Work out the finished part from the listing and answer in its coordinate system (mm). Give positions to 0.01 mm unless a question says otherwise; leave off trailing zeros. Order: outer loops, then holes, each group sorted by start corner. A loop starts at its lowest first (then second) coordinate and runs counter-clockwise, first axis right, second up. Notation, with made-up numbers: (-4.75, -30) - (41.25, -30) arc R26 cw to (41.25, -7) - close; hole circle Ø3 at (78.5, 86). An arc over 180 degrees is marked (long way). Return JSON: item names as keys, results as strings. Group by question number.
from build123d import *

# Parameters (mm, degrees)
F0_R     = 2.49938
F1_DEPTH = 101.6


with BuildPart() as f1:
    # F0 (on Front) → F1 (new body)
    with BuildSketch(Plane.XZ):
        with BuildLine():
            ThreePointArc((-24.424371, 19.05), (-45.903919, 14.384096), (-62.524371, 0))
            Line((-62.524371, 0), (-24.424371, 0))
            Line((-24.424371, 0), (28.877782, 0))
            Line((28.877782, 0), (28.877782, 33.381656))
            ThreePointArc((28.877782, 33.381656), (2.940295, 23.561851), (-24.424371, 19.05))
        make_face()
        with Locations((-45.833543, 4.23894)):
            Circle(F0_R, mode=Mode.SUBTRACT)
    extrude(amount=F1_DEPTH)


solid = f1.part
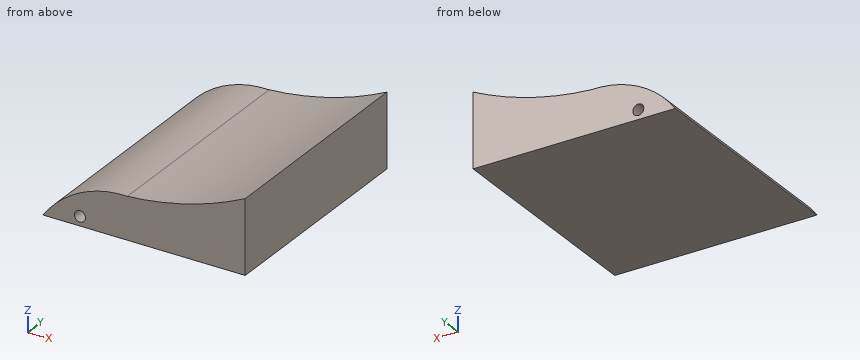
1. The part is cut by section A-A (y = -38). Give the vertices of the cut face in (x, z), and give its area (3 significant figures).
2. This flat-tipped pin is pushed along its axis until it touches: pin 1 (5 mm diameter, centred on x = -49.5, z = 13.5, fed in from +Y). Where does it stop, or does it pass through?
3. Consider probe 1 along Z at (x, y) = (-45, -18.5); probe 2 along X at (y, z) = (-39.5, 5.5); probe 3 along Z at (x, y) = (25.5, -51.5). Determine where each line is inside the solid, lowest interval first. Write a range as from..to.
4. The part is cut by section C-C (x = -54). Give the vertices of the cut face in (y, z).
5. The part is cut by section B-B (z = 29.5). Give the vertices of the cut face in (x, y).
Answers:
{
 "1": {"outline": "(-62.52, 0) - (28.88, 0) - (28.88, 33.38) arc R139.94 cw to (-24.42, 19.05) arc R44.47 ccw to start; hole circle Ø5 at (-45.83, 4.24)", "area": "1,800 mm^2"},
 "2": {"pin 1": "stops at y = 0"},
 "3": {"probe 1": "z = 0..1.88, 6.6..14.82", "probe 2": "x = -58.01..-47.99, -43.68..28.88", "probe 3": "z = 0..31.76"},
 "4": {"outline": "(-101.6, 0) - (0, 0) - (0, 9.17) - (-101.6, 9.17) - close"},
 "5": {"outline": "(20.36, -101.6) - (28.88, -101.6) - (28.88, 0) - (20.36, 0) - close"}
}
